Autodesk Inventor part; units mm, degrees
ref_plane "YZ Plane" through (0, 0, 0) normal (1, 0, 0) x (0, 1, 0)
ref_plane "XZ Plane" through (0, 0, 0) normal (0, 1, 0) x (-1, 0, 0)
ref_plane "XY Plane" through (0, 0, 0) normal (0, 0, 1) x (1, 0, 0)
sketch "Sketch1" plane through (0, 0, 0) normal (0, 1, 0) x (-1, 0, 0)
  line L0 (6.3007, 16.0107) -> (6.8999, 16.0107)
  line L1 (3.7249, 12.8357) -> (3.7249, -5.8651)
  line L2 (6.8999, -9.0401) -> (6.3007, -9.0401)
  line L3 (9.4757, -5.8651) -> (9.4757, 12.8357)
  arc A0 (9.4757, 12.8357) -> (6.3007, 16.0107) centre (6.3007, 12.8357) ccw
  arc A1 (6.3007, -9.0401) -> (9.4757, -5.8651) centre (6.3007, -5.8651) ccw
  arc A2 (3.7249, -5.8651) -> (6.8999, -9.0401) centre (6.8999, -5.8651) ccw
  arc A3 (6.8999, 16.0107) -> (3.7249, 12.8357) centre (6.8999, 12.8357) ccw
  circle A4 centre (6.6003, 12.8357) radius 1.745
  circle A5 centre (6.6003, -5.8651) radius 1.5248
  point P0 (0, 0)
  point P1 (6.6003, 15.9965)
  point P2 (6.6003, -9.0259)
  dimension "d0" = 3.175
extrude "Extrusion1" add sketch "Sketch1" along normal blind 2.54 contours A0 L3 A1 A2 L1 A3
properties part number "GRIPPER1"
Source: CAD feature listing. Evaluate the final solid. Frame: model axes, mm. Round coordinates to 2 decimals unless told otherwise and drop trailing zeros. Order: outer loops, then holes, each group sorted by start corner. A loop starts at its lowest first (then second) coordinate and runs counter-clockwise, first axis right, second up. Notation, with made-up numbers: (37.25, -7) - (64.25, -7) arc R27 ccw to (64.25, 11) - close; hole circle Ø11 at (-10, -34.5). An arc over 180 degrees is marked (long way). Use a Markdown table: item, result. Add a question column.
1. Section query A-A (y = 1.8). Return the cut outline in (x, z) (3 decimals), then the cut area to 3 significant figures.
2. Mould query, pull axis Z, two halves, no side actions, for faces 1 (the cylindrical face through (-8.627, 1.252, 14.996)), 2 (the cylindrical face through (-8.01, 1.25, -5.28)), 3 (the flat face through (-7, 2.54, 4)). Classes: +Z half, -Z half, draft (parallel to the pull), parting line (faces both ways), or undercut.
3. First-contact query: pin 1 (1 mm diameter, centred on x = -7.5, y = 2, fed in from -Z). Flat tip, straight axial feed; report the tip coordinate or a pass-through.
4. Section query B-B (z = -5). Return the cut outline in (x, y), then the cut area to 3 significant figures.
5. Section query C-C (x = -7.15). Return the cut outline in (y, z) (3 decimals).
6. Line query: probe 1 along Z at (x, y) = (-7.45, 0.45); probe 2 along X at (y, z) = (1.15, -6); probe 3 along X at (y, z) = (0.5, 11.5). Output: solid intervals per line, ascending.
7. Section query D-D (x = -9). Return the cut outline in (y, z), then the cut area to 3 significant figures.
Derived:
| question | item | result |
|---|---|---|
| 1 | outline | (-9.476, -5.865) arc R3.175 ccw to (-6.6, -9.026) arc R3.175 ccw to (-3.725, -5.865) - (-3.725, 12.836) arc R3.175 ccw to (-6.6, 15.997) arc R3.175 ccw to (-9.476, 12.836) - close; hole circle Ø3.49 at (-6.6, 12.836); hole circle Ø3.05 at (-6.6, -5.865) |
| 1 | area | 119 mm2 |
| 2 | face 1 | +Z half |
| 2 | face 2 | undercut |
| 2 | face 3 | draft |
| 3 | pin 1 | z = -8.96 |
| 4 | outline | (-9.48, 0) - (-7.86, 0) - (-7.86, 2.54) - (-9.48, 2.54) - close; (-5.34, 0) - (-3.72, 0) - (-3.72, 2.54) - (-5.34, 2.54) - close |
| 4 | area | 8.23 mm2 |
| 5 | outline | (0, -8.924) - (2.54, -8.924) - (2.54, -7.287) - (0, -7.287) - close; (0, -4.443) - (2.54, -4.443) - (2.54, 11.18) - (0, 11.18) - close; (0, 14.492) - (2.54, 14.492) - (2.54, 15.895) - (0, 15.895) - close |
| 6 | probe 1 | -8.82 to -7.13, -4.6 to 11.31, 14.36 to 15.8 |
| 6 | probe 2 | -9.47 to -8.12, -5.08 to -3.73 |
| 6 | probe 3 | -9.48 to -7.72, -5.48 to -3.72 |
| 7 | outline | (0, -7.54) - (2.54, -7.54) - (2.54, 14.51) - (0, 14.51) - close |
| 7 | area | 56.0 mm2 |
